Model file for the job. Use its own axes, mm. A direction names the side the tool comes from. Coordinates: 2 decimals unless noted, no trailing zeros. Loops run counter-clockwise (first coordinate to the right, second up) from the corner with the lowest first, then second, coordinate; pieces in that order, holes last. Notation, with made-up numbers: M -22.5,-34.5 L -1.5,-34.5 A28 ccw -1.5,1.5 Z; hole C 43,-35 d5. An arc over 180 degrees is marked long. Write item = value, one per line. Start each with the question number.
from build123d import *

# Parameters (mm, degrees)
BOSS_EXTRUDE1_DEPTH = 1.6


with BuildPart() as part:
    # Sketch1 → Boss-Extrude1 (new body)
    with BuildSketch(Plane(origin=(0, 0, 0), x_dir=(1, 0, 0), z_dir=(0, 1, 0))):
        with BuildLine():
            Line((623.01202177, -61.448413556), (625.01202177, -61.448413556))
            ThreePointArc((625.01202177, -61.448413556), (625.36557516, -61.301966947), (625.51202177, -60.948413556))
            Line((625.51202177, -60.948413556), (625.51202177, -40.948413556))
            ThreePointArc((625.51202177, -40.948413556), (625.36557516, -40.594860166), (625.01202177, -40.448413556))
            Line((625.01202177, -40.448413556), (618.76202177, -40.448413556))
            Line((618.76202177, -40.448413556), (618.51202177, -40.448413556))
            Line((618.51202177, -40.448413556), (618.51202177, -48.548413556))
            Line((618.51202177, -48.548413556), (616.51202177, -48.548413556))
            Line((616.51202177, -48.548413556), (616.51202177, -40.448413556))
            Line((616.51202177, -40.448413556), (616.26202177, -40.448413556))
            Line((616.26202177, -40.448413556), (616.01202177, -40.448413556))
            ThreePointArc((616.01202177, -40.448413556), (615.658468379, -40.594860166), (615.51202177, -40.948413556))
            Line((615.51202177, -40.948413556), (615.51202177, -58.448413556))
            Line((615.51202177, -58.448413556), (616.26202177, -58.448413556))
            Line((616.26202177, -58.448413556), (618.76202177, -58.448413556))
            Line((618.76202177, -58.448413556), (622.51202177, -58.448413556))
            Line((622.51202177, -58.448413556), (622.51202177, -60.948413556))
            ThreePointArc((622.51202177, -60.948413556), (622.658468379, -61.301966947), (623.01202177, -61.448413556))
        make_face()
    extrude(amount=BOSS_EXTRUDE1_DEPTH)


solid = part.part
Item 1: Pin check, flat tips, straight feed: pin 1 Ø0.8 at (x, y) = (619, 1) entering from +Z; pin 2 Ø0.5 at (y, z) = (1, 60) entering from -X. Stop position of each tip, or through.
Item 2: Cut at C-C (z = 59.25). Give the cut face in (x, y), plus the area to 3 significant figures.
Item 3: 3-axis set-ups, long thin cutter, end or side, ignore diameter. For faces 5 (the flat face through (620, 1.6, 51)), 6 (the flat face through (616.512, 1, 45)), 7 (the flat face through (619, 1, 58.448)): which of +Z, -Z, +X, -X, +Y, -Y reach the whole face in a straight line?
Item 4: Pull direction X, two halves, no side cores. Call faces 1 (the flat face through (618.512, 1, 44)), 2 (the flat face through (615.512, 1, 50)), 3 (the flat face through (624, 1, 61.448)), 4 (the flat face through (625.512, 1, 51)): +X half, -X half, draft (parallel to the pull), parting line (faces both ways), or undercut.
Item 5: Cut at B-B (y = 0.25). Give the cut face in (x, z), plus the area to 3 significant figures.
Item 6: Probe L1, parallel to X at y = 0.3, z = 46.25; L2, parallel to Z at x = 621.75, y = 1.5; L3, parallel to X at y = 1.45, z = 60.75. List the from-to ranges inside material, lowest first.
Item 7: Cut at D-D (x = 620.75). Give the cut face in (y, z).
Item 8: Cut at A-A (z = 46.5). Give the cut face in (x, y), plus the area to 3 significant figures.
Reported:
q1.pin_1 = 58.45
q1.pin_2 = 622.51
q2.outline = M 622.51,0 L 625.51,0 L 625.51,1.6 L 622.51,1.6 Z
q2.area = 4.80 mm^2
q3.face_5 = +Z, -Z, +X, -X, +Y
q3.face_6 = -Z, +Y, -Y
q3.face_7 = +Z, -X, +Y, -Y
q4.face_1 = undercut
q4.face_2 = -X half
q4.face_3 = draft
q4.face_4 = +X half
q5.outline = M 615.51,40.95 A0.5 ccw 616.01,40.45 L 616.51,40.45 L 616.51,48.55 L 618.51,48.55 L 618.51,40.45 L 625.01,40.45 A0.5 ccw 625.51,40.95 L 625.51,60.95 A0.5 ccw 625.01,61.45 L 623.01,61.45 A0.5 ccw 622.51,60.95 L 622.51,58.45 L 615.51,58.45 Z
q5.area = 173 mm^2
q6.L1 = 615.51 to 616.51, 618.51 to 625.51
q6.L2 = 40.45 to 58.45
q6.L3 = 622.51 to 625.51
q7.outline = M 0,40.45 L 1.6,40.45 L 1.6,58.45 L 0,58.45 Z
q8.outline = M 615.51,0 L 616.51,0 L 616.51,1.6 L 615.51,1.6 Z; M 618.51,0 L 625.51,0 L 625.51,1.6 L 618.51,1.6 Z
q8.area = 12.8 mm^2
